Can you work these out from the model? Positions are in its coordinate system, mm. Coordinates: 2 decimals unless noted, no trailing zeros. Write each loop counter-clockwise with the first axis right and the second up, starting at its lowest first coordinate (ties: lowest second). Pieces come first, ordered by that corner, then holes. Notation, with made-up numbers: (55.25, 64.25) -> (99.25, 64.25) arc R25 ccw to (99.25, 93.25) -> close; hole circle Ø9 at (86, 67.5). An arc over 180 degrees is marked (long way). Answer as CSV lines item,"result". Start each with the question number.
```python
from build123d import *

# Parameters (mm, degrees)
SKETCH_1_R          = 1.55
EXTRUDE_1_DEPTH     = 2
SKETCH_2_R          = 1.55
CUT_EXTRUDE_1_DEPTH = 3
SKETCH_4_R          = 2.5
CUT_EXTRUDE_2_DEPTH = 3


with BuildPart() as part:
    # 草图1 → 凸台-拉伸1 (new body)
    with BuildSketch(Plane.XY):
        with BuildLine():
            Line((-2.598076211, 21.5), (-19.918584287, -8.5))
            ThreePointArc((-19.918584287, -8.5), (-19.918584287, -11.5), (-17.320508076, -13))
            Line((-17.320508076, -13), (17.320508076, -13))
            ThreePointArc((17.320508076, -13), (19.918584287, -11.5), (19.918584287, -8.5))
            Line((19.918584287, -8.5), (2.598076211, 21.5))
            ThreePointArc((2.598076211, 21.5), (0, 23), (-2.598076211, 21.5))
        make_face()
        with Locations((0, 20)):
            Circle(SKETCH_1_R, mode=Mode.SUBTRACT)
        with Locations((17.320508076, -10)):
            Circle(SKETCH_1_R, mode=Mode.SUBTRACT)
        with Locations((-17.320508076, -10)):
            Circle(SKETCH_1_R, mode=Mode.SUBTRACT)
    extrude(amount=EXTRUDE_1_DEPTH)

    # 草图2 → 切除-拉伸1 (cut)
    with BuildSketch(Plane.XY.offset(2)):
        with Locations((0, 6)):
            Circle(SKETCH_2_R)
        with Locations((6, 0)):
            Circle(SKETCH_2_R)
        with Locations((0, -6)):
            Circle(SKETCH_2_R)
        with Locations((-6, 0)):
            Circle(SKETCH_2_R)
    extrude(amount=-CUT_EXTRUDE_1_DEPTH, mode=Mode.SUBTRACT)

    # 草图4 → 切除-拉伸2 (cut)
    with BuildSketch(Plane.XY.offset(2)):
        Circle(SKETCH_4_R)
    extrude(amount=-CUT_EXTRUDE_2_DEPTH, mode=Mode.SUBTRACT)


solid = part.part
```
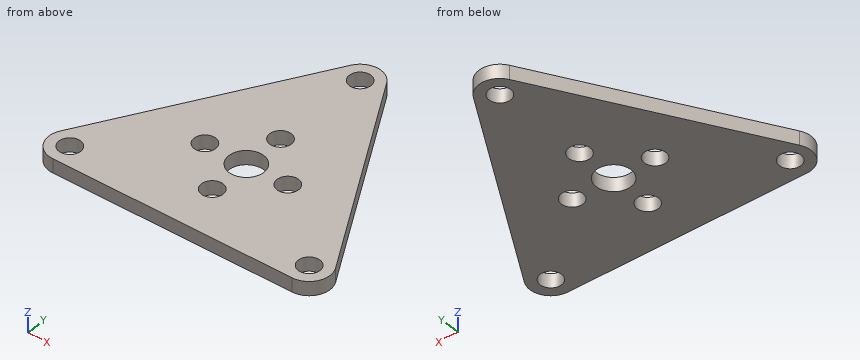
Q1. Imagine slicing it at D-D (y = -2). Write out the boundary of the cut face in (x, z).
Q2. Imagine slicing it at B-B (x = 0). Write out the boundary of the cut face in (y, z).
Q3. Imagine slicing it at C-C (z = 0.65). State how many separate pieces and enclosed holes the cut face has, then the cut area to 3 significant figures.
Q4. Imagine slicing it at A-A (y = -10). Write out the boundary of the cut face in (x, z).
Q5. I need wall thicknesses on L1, parallel to Y at x = 0, z = 1.45; L2, parallel to Y at x = 7, z = 0.85; L3, parallel to X at y = 21, z = 1.3. Which ranges of each line are inside material? Lowest first, please.
Entries:
1,outline,"(-16.17, 0) -> (-1.5, 0) -> (-1.5, 2) -> (-16.17, 2) -> close; (1.5, 0) -> (16.17, 0) -> (16.17, 2) -> (1.5, 2) -> close"
2,outline,"(-13, 0) -> (-7.55, 0) -> (-7.55, 2) -> (-13, 2) -> close; (-4.45, 0) -> (-2.5, 0) -> (-2.5, 2) -> (-4.45, 2) -> close; (2.5, 0) -> (4.45, 0) -> (4.45, 2) -> (2.5, 2) -> close; (7.55, 0) -> (18.45, 0) -> (18.45, 2) -> (7.55, 2) -> close; (21.55, 0) -> (23, 0) -> (23, 2) -> (21.55, 2) -> close"
3,separate pieces,"1"
3,enclosed holes,"8"
3,area,"787 mm2"
4,outline,"(-20.32, 0) -> (-18.87, 0) -> (-18.87, 2) -> (-20.32, 2) -> close; (-15.77, 0) -> (15.77, 0) -> (15.77, 2) -> (-15.77, 2) -> close; (18.87, 0) -> (20.32, 0) -> (20.32, 2) -> (18.87, 2) -> close"
5,L1,"-13 to -7.55, -4.45 to -2.5, 2.5 to 4.45, 7.55 to 18.45, 21.55 to 23"
5,L2,"-13 to -1.18, 1.18 to 13.88"
5,L3,"-2.89 to -1.18, 1.18 to 2.89"
